For this review, use the dimensioned drawing (mm, ordinates from the lowest corner) and the shaded views. A direction names the side the tool comes from. Give positions to 0.01 mm unless a question says otherwise; leave off trailing zeros. Write each loop counter-clockwise with the first axis right and the second up, starting at its lowest first coordinate (ties: lowest second). Pieces come first, ordered by that corner, then holes. Notation, with made-up numbers: M 30,-39 L 45,-39 A15 ccw 45,-13 Z; hole C -15,-2 d9. An arc over 180 degrees is marked long. Answer in a Markdown table with one row per item.
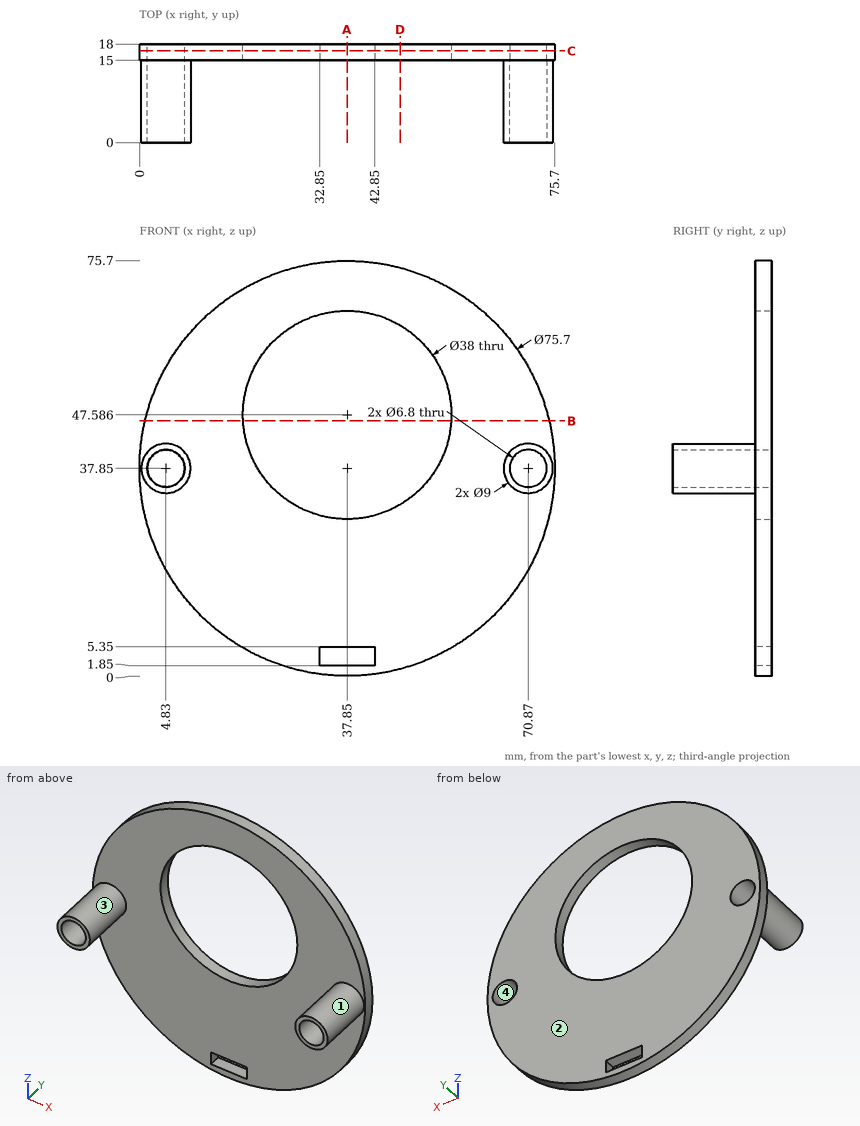
1) To check wall thickness, follow probe 1 along Z at (x, y) = (37.85, 15.7); probe 2 along Z at (x, y) = (4.83, 8.5); probe 3 along Z at (x, y) = (33.5, 15.25). State the ranges of each line that lie inside material, in increasing order. Write a range as [from, to].
Geometry says:
| item | result |
|---|---|
| probe 1 | [0, 1.85], [5.35, 28.59], [66.59, 75.7] |
| probe 2 | [33.35, 34.45], [41.25, 42.35] |
| probe 3 | [0.25, 1.85], [5.35, 29.09], [66.08, 75.45] |
2) The part is to be moulded in two halves that separate along X. For the marked faces 1 and 2, say which applies: released by +X, released by -X, zero draft, split by the parting line, or undercut.
Geometry says:
| item | result |
|---|---|
| face 1 | undercut |
| face 2 | zero draft |
3) Add section A-A (x = 37.85). Write out the cut boundary in (y, z).
Geometry says:
| item | result |
|---|---|
| outline | M 15,0 L 18,0 L 18,1.85 L 15,1.85 Z; M 15,5.35 L 18,5.35 L 18,28.59 L 15,28.59 Z; M 15,66.59 L 18,66.59 L 18,75.7 L 15,75.7 Z |
4) Add section B-B (z = 46.5). Write out the cut boundary in (x, y).
Geometry says:
| item | result |
|---|---|
| outline | M 1,15 L 18.88,15 L 18.88,18 L 1,18 Z; M 56.82,15 L 74.7,15 L 74.7,18 L 56.82,18 Z |
5) Add section C-C (y = 16.75). Write out the cut boundary in (x, z), and give its area (3 significant figures).
Geometry says:
| item | result |
|---|---|
| outline | C 37.85,37.85 d75.7; hole C 4.83,37.85 d6.8; hole C 37.85,47.59 d38; hole M 32.85,1.85 L 42.85,1.85 L 42.85,5.35 L 32.85,5.35 Z; hole C 70.87,37.85 d6.8 |
| area | 3,260 mm^2 |
6) For the marked faces 3 and 4, list the 3-axis set-ups (+Z, -Z, +X, -X, +Y, -Y) from which the entire face can be reached by the end or side of a thin tool; tool diameter is ignored.
Geometry says:
| item | result |
|---|---|
| face 3 | -Y |
| face 4 | +Y, -Y |
7) Insertion check: P1, Ø1.5, axis at x = 52, z = 28.5, coming from the -Y side; P2, Ø8, axis at y = 3, z = 37, coming from the +X side; P3, Ø10, axis at x = 21, y = 14, coming from the +Z side. Each pin has a flat end and moves straight along its axis. Give the tip position at first contact, or say it passes through.
Geometry says:
| item | result |
|---|---|
| P1 | y = 15 |
| P2 | x = 75.37 |
| P3 | z = 73.76 |
8) Add section D-D (x = 47.5). Write out the cut boundary in (y, z).
Geometry says:
| item | result |
|---|---|
| outline | M 15,1.25 L 18,1.25 L 18,31.22 L 15,31.22 Z; M 15,63.95 L 18,63.95 L 18,74.45 L 15,74.45 Z |
